Could you check a few things on this model? Use its own coordinates, in mm. A direction names the side the tool comes from. Give positions to 0.01 mm unless a question says otherwise; leave off trailing zeros. Order: outer loops, then holes, each group sorted by start corner. A loop starts at its lowest first (then second) coordinate and runs counter-clockwise, first axis right, second up. Notation, with made-up numbers: (85.5, -32.5) - (102.5, -32.5) arc R33 ccw to (102.5, -0.5) - close; hole circle Ø4 at (40, 45). An arc over 180 degrees is marked (long way). Put each result on its own line as item: value.
from build123d import *

# Parameters (mm, degrees)
SKETCH1_W           = 114.3
SKETCH1_H           = 40.64
BOSS_EXTRUDE1_DEPTH = 2.54
SKETCH2_R           = 1.5875
CUT_EXTRUDE2_DEPTH  = 61.708125486
SKETCH3_W           = 43.201910461
SKETCH3_H           = 17.373570515
SKETCH3_W_2         = 46.628586193
SKETCH3_H_2         = 22.401940477
CUT_EXTRUDE3_DEPTH  = 61.708125486
SKETCH4_W           = 2.643760601
SKETCH4_H           = 17.553517305
BOSS_EXTRUDE2_DEPTH = 7.62
SKETCH5_W           = 17.553517305
SKETCH5_H           = 2.255880329
BOSS_EXTRUDE3_DEPTH = 33.782
BOSS_EXTRUDE4_DEPTH = 2.54


with BuildPart() as part:
    # Sketch1 → Boss-Extrude1 (new body)
    with BuildSketch(Plane(origin=(0, 0, 0), x_dir=(1, 0, 0), z_dir=(0, 1, 0))):
        Rectangle(SKETCH1_W, SKETCH1_H)
    extrude(amount=BOSS_EXTRUDE1_DEPTH)

    # Sketch2 → Cut-Extrude2 (cut, through all)
    with BuildSketch(Plane(origin=(0, 2.54, 0), x_dir=(1, 0, 0), z_dir=(0, 1, 0))):
        with Locations(Location((-52.07, 16.51, 0), (0, 0, 270))):
            Circle(SKETCH2_R)
        with Locations(Location((52.07, 16.51, 0), (0, 0, 270))):
            Circle(SKETCH2_R)
        with Locations(Location((52.07, -16.51, 0), (0, 0, 270))):
            Circle(SKETCH2_R)
        with Locations(Location((-52.07, -16.51, 0), (0, 0, 270))):
            Circle(SKETCH2_R)
    extrude(amount=-CUT_EXTRUDE2_DEPTH, mode=Mode.SUBTRACT)

    # Sketch3 → Cut-Extrude3 (cut, through all)
    with BuildSketch(Plane(origin=(0, 2.54, 0), x_dir=(1, 0, 0), z_dir=(0, 1, 0))):
        with Locations((37.284400117, -0.013259404)):
            Rectangle(SKETCH3_W, SKETCH3_H)
        with Locations((-20.818521539, 19.874496091)):
            Rectangle(SKETCH3_W_2, SKETCH3_H_2)
    extrude(amount=-CUT_EXTRUDE3_DEPTH, mode=Mode.SUBTRACT)

    # Sketch4 → Boss-Extrude2 (add)
    with BuildSketch(Plane(origin=(0, 2.54, 0), x_dir=(1, 0, 0), z_dir=(0, 1, 0))):
        with Locations((14.361564587, -0.103232799)):
            Rectangle(SKETCH4_W, SKETCH4_H)
    extrude(amount=BOSS_EXTRUDE2_DEPTH)

    # Sketch5 → Boss-Extrude3 (add)
    with BuildSketch(Plane(origin=(15.683444887, 0, 0), x_dir=(0, 0, -1), z_dir=(1, 0, 0))):
        with Locations((-0.103232799, 9.032059836)):
            Rectangle(SKETCH5_W, SKETCH5_H)
    extrude(amount=BOSS_EXTRUDE3_DEPTH)

    # Sketch6 → Boss-Extrude4 (add)
    with BuildSketch(Plane(origin=(0, 2.54, 0), x_dir=(1, 0, 0), z_dir=(0, 1, 0))):
        Polygon((57.15, 20.32), (57.15, 8.673525853), (62.36601956, 8.673525853), (62.36601956, -9.230657654), (57.15, -9.230657654), (57.15, -20.32), (67.276494875, -20.32), (67.276494875, 20.32), align=None)
    extrude(amount=-BOSS_EXTRUDE4_DEPTH)


solid = part.part
1) Suppose I cut it at B-B, the plane x = -52.07. List the corners of the cut face in (y, z) for me.
Filled in:
outline: (0, -20.32) - (2.54, -20.32) - (2.54, -18.1) - (0, -18.1) - close; (0, -14.92) - (2.54, -14.92) - (2.54, 14.92) - (0, 14.92) - close; (0, 18.1) - (2.54, 18.1) - (2.54, 20.32) - (0, 20.32) - close
2) We'd pull the mould along Z, two halves only. Please class faces 1 (the flat face through (-51, 1, -20.32)), 2 (the flat face through (67.276, 1, 0)), 3 (the flat face through (36, 1, 8.7)): pulls with the +Z half, pulls with the -Z half, needs draft (parallel to the pull), parting line crosses it, or undercut.
Filled in:
face 1: pulls with the -Z half
face 2: needs draft
face 3: undercut
3) Suppose I cut it at A-A, the plane z = -16.51. List the corners of the cut face in (x, y) for me, and give its area (3 significant figures).
Filled in:
outline: (-57.15, 0) - (-53.66, 0) - (-53.66, 2.54) - (-57.15, 2.54) - close; (-50.48, 0) - (-44.13, 0) - (-44.13, 2.54) - (-50.48, 2.54) - close; (2.5, 0) - (50.48, 0) - (50.48, 2.54) - (2.5, 2.54) - close; (53.66, 0) - (67.28, 0) - (67.28, 2.54) - (53.66, 2.54) - close
area: 181 mm^2
4) I'm going to push flat-ended pins straight in: pin 1 (20.5 mm diameter, centred on x = 2, z = -2, fed in from +Y); pin 2 (3.5 mm diameter, centred on x = -52.07, z = 16.51, fed in from -Y); pin 3 (4 mm diameter, centred on y = 5, z = 11.5, fed in from +X); pin 4 (1.3 mm diameter, centred on x = -13, y = 0.5, fed in from -Z). Where does each tip first touch, or does it pass through?
Filled in:
pin 1: stops at y = 2.54
pin 2: stops at y = 0
pin 3: passes through
pin 4: stops at z = -8.67
5) Suppose I cut it at C-C, the plane z = -6.5. List the corners of the cut face in (x, y) for me.
Filled in:
outline: (-57.15, 0) - (15.68, 0) - (15.68, 7.9) - (49.47, 7.9) - (49.47, 10.16) - (13.04, 10.16) - (13.04, 2.54) - (-57.15, 2.54) - close; (62.37, 0) - (67.28, 0) - (67.28, 2.54) - (62.37, 2.54) - close
6) Suppose I cut it at D-D, the plane x = 52.07. List the corners of the cut face in (y, z) for me.
Filled in:
outline: (0, -20.32) - (2.54, -20.32) - (2.54, -18.1) - (0, -18.1) - close; (0, -14.92) - (2.54, -14.92) - (2.54, -8.67) - (0, -8.67) - close; (0, 8.7) - (2.54, 8.7) - (2.54, 14.92) - (0, 14.92) - close; (0, 18.1) - (2.54, 18.1) - (2.54, 20.32) - (0, 20.32) - close
7) Which directions (+Z, -Z, +X, -X, +Y, -Y) give clear straight access to the entire face, cutting with the end or side of a thin tool? Please do faces 4 (the flat face through (60, 1, 9.231)), 5 (the flat face through (-44.133, 1, -14)), 6 (the flat face through (13.04, 6, 0)), 7 (the flat face through (27, 9, 8.88)).
Filled in:
face 4: +Y, -Y
face 5: -Z, +Y, -Y
face 6: +Z, -Z, -X, +Y
face 7: +Z, +X, -X, +Y
8) If I drill on line 1 (X direction, y = 1.8, z = -16.51); line 2 (Z direction, x = -52, y = 2.5); line 3 (X direction, y = 1.6, z = 16.51), over which ranges is the centre line in solid material (lowest first)? Write a range as [from, to].
Filled in:
line 1: x = [-57.15, -53.66], [-50.48, -44.13], [2.5, 50.48], [53.66, 67.28]
line 2: z = [-20.32, -18.1], [-14.92, 14.92], [18.1, 20.32]
line 3: x = [-57.15, -53.66], [-50.48, 50.48], [53.66, 67.28]
